Build history of the part. All positions in model axes, mm. A direction names the side the tool comes from. Round coordinates to 2 decimals unless told otherwise and drop trailing zeros. Write each loop counter-clockwise with the first axis right and the second up, starting at its lowest first coordinate (ties: lowest second). Pieces come first, ordered by that corner, then holes.
from build123d import *

# Parameters (mm, degrees)
F0_W     = 13
F0_H     = 13
F0_W_2   = 0.225
F0_H_2   = 1
F1_DEPTH = 10
F2_DEPTH = 0.4


with BuildPart() as f1:
    # F0 (on Top) → F1 (new body)
    with BuildSketch(Plane.XY):
        with Locations((-3.3, 3.3)):
            Rectangle(F0_W, F0_H)
        Polygon((-6.825, 2.8), (-6.825, 3.8), (-6.825, 6.825), (0.225, 6.825), (0.225, 3.8), (0.225, 2.8), (0.225, -0.225), (-6.825, -0.225), align=None, mode=Mode.SUBTRACT)
        with Locations((0.1125, 3.3)):
            Rectangle(F0_W_2, F0_H_2)
        with Locations((-6.7125, 3.3)):
            Rectangle(F0_W_2, F0_H_2)
    extrude(amount=F1_DEPTH)

    # F0 (on Top) → F2 (join)
    with BuildSketch(Plane.XY):
        Polygon((-6.6, 0), (-6.6, 2.8), (-6.825, 2.8), (-6.825, -0.225), (0.225, -0.225), (0.225, 2.8), (0, 2.8), (0, 0), align=None)
        Polygon((-6.6, 3.8), (-6.6, 6.6), (0, 6.6), (0, 3.8), (0.225, 3.8), (0.225, 6.825), (-6.825, 6.825), (-6.825, 3.8), align=None)
    extrude(amount=F2_DEPTH)


solid = f1.part
1) Wall check: L1, parallel to Y at x = -1.25, z = 2 (3 decimals); L2, parallel to X at y = 4.75, z = 0.5 (3 decimals); L3, parallel to X at y = 3.5, z = 7. Give the ranges that are in metal, low to high.
Results:
L1: y = -3.2 to -0.225, 6.825 to 9.8
L2: x = -9.8 to -6.825, 0.225 to 3.2
L3: x = -9.8 to -6.6, 0 to 3.2
2) Mould opens along X. For faces 4 (the flat face through (-3, -1, 10)), 5 (the flat face through (-9.8, 3, 5)), 6 (the flat face through (0.225, 1, 5)) say: released by +X, released by -X, zero draft, split by the parting line, or undercut.
Results:
face 4: zero draft
face 5: released by -X
face 6: undercut
3) Slice it at A-A (z = 7.75). Write the cut outline in (x, y) (3 decimals).
Results:
outline: (-9.8, -3.2) - (3.2, -3.2) - (3.2, 9.8) - (-9.8, 9.8) - close; hole (-6.825, -0.225) - (0.225, -0.225) - (0.225, 2.8) - (0, 2.8) - (0, 3.8) - (0.225, 3.8) - (0.225, 6.825) - (-6.825, 6.825) - (-6.825, 3.8) - (-6.6, 3.8) - (-6.6, 2.8) - (-6.825, 2.8) - close
4) Slice it at B-B (y = 4). Write the cut outline in (x, z) (3 decimals).
Results:
outline: (-9.8, 0) - (-6.6, 0) - (-6.6, 0.4) - (-6.825, 0.4) - (-6.825, 10) - (-9.8, 10) - close; (0, 0) - (3.2, 0) - (3.2, 10) - (0.225, 10) - (0.225, 0.4) - (0, 0.4) - close
5) Which spindle directions (+Z, -Z, +X, -X, +Y, -Y) get a long thin tool onto all of the face, cutting with end or side? Do faces 1 (the flat face through (-6.825, 1, 5)), 2 (the flat face through (0, 3, 4)), 3 (the flat face through (-3, -3.2, 5)). Say none if no direction does.
Results:
face 1: +Z
face 2: +Z, -Z
face 3: +Z, -Z, +X, -X, -Y
6) Slice it at C-C (x = -2.5). Write the cut outline in (y, z) (3 decimals), plus the area to 3 significant figures.
Results:
outline: (-3.2, 0) - (0, 0) - (0, 0.4) - (-0.225, 0.4) - (-0.225, 10) - (-3.2, 10) - close; (6.6, 0) - (9.8, 0) - (9.8, 10) - (6.825, 10) - (6.825, 0.4) - (6.6, 0.4) - close
area: 59.7 mm2
